Build history of the part. All positions in model axes, mm. Face numbers are marked on the shaded views. A direction names the side the tool comes from. Give positions to 0.01 mm unless a question says otherwise; leave off trailing zeros. Order: outer loops, then holes, each group sorted by start corner. A loop starts at its lowest first (then second) coordinate and runs counter-clockwise, first axis right, second up. Notation, with made-up numbers: (35, 86.5) - (43, 86.5) arc R26 ccw to (43, 123.5) - close; hole circle Ø10 at (-37, -28.5). An arc over 180 degrees is marked (long way). Answer in a Markdown table with one row per item.
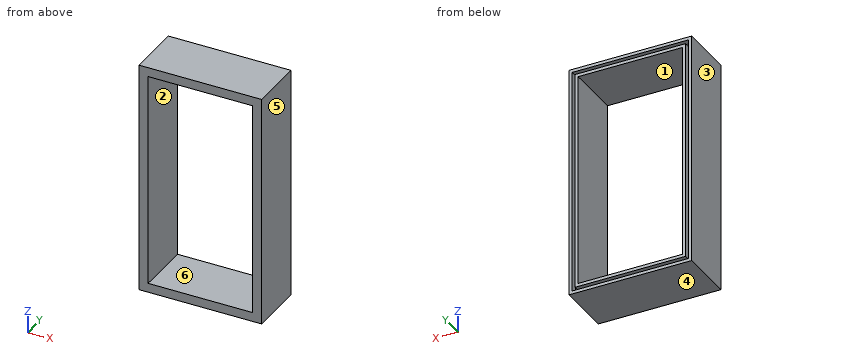
Autodesk Inventor part; units mm, degrees
ref_plane "Work Plane1" through (508, 0, 0) normal (1, 0, 0) x (0, 0, -1)
ref_plane "Work Plane2" through (1016, 0, -965.2) normal (0, 0, -1) x (-1, 0, 0)
ref_plane "YZ Plane" through (0, 0, 0) normal (1, 0, 0) x (0, 1, 0)
sketch "Sketch1" plane through (0, 0, 0) normal (0, 1, 0) x (-1, 0, 0)
  line L0 (0, 0) -> (-1016, 0)
  line L1 (-1016, 0) -> (-1016, -1930.4)
  line L2 (-1016, -1930.4) -> (0, -1930.4)
  line L3 (0, -1930.4) -> (0, 0)
  dimension "d0" = 1016
  dimension "d1" = 1930.4
extrude "Extrusion1" add sketch "Sketch1" along normal blind 457.2
sketch "Sketch8" plane through (0, 457.2, 0) normal (0, 1, 0) x (1, 0, 0)
  line L0 (25.4, 25.4) -> (990.6, 25.4)
  line L1 (990.6, 25.4) -> (990.6, 1905)
  line L2 (990.6, 1905) -> (25.4, 1905)
  line L3 (25.4, 1905) -> (25.4, 25.4)
  line L4 (50.8, 50.8) -> (965.2, 50.8)
  line L5 (965.2, 50.8) -> (965.2, 1879.6)
  line L6 (965.2, 1879.6) -> (50.8, 1879.6)
  line L7 (50.8, 1879.6) -> (50.8, 50.8)
  line L8 (50.8, 965.2) -> (25.4, 965.2)
  line L9 (965.2, 965.2) -> (990.6, 965.2)
  line L10 (508, 1879.6) -> (508, 1905)
  line L11 (508, 50.8) -> (508, 25.4)
  line L12 (508, 25.4) -> (508, 0)
  line L13 (0, 0) -> (1016, 0)
  line L14 (508, 1905) -> (508, 1930.4)
  line L15 (1016, 1930.4) -> (0, 1930.4)
  line L16 (25.4, 965.2) -> (0, 965.2)
  line L17 (0, 1930.4) -> (0, 0)
  line L18 (990.6, 965.2) -> (1016, 965.2)
  line L19 (1016, 0) -> (1016, 1930.4)
  dimension "d13" = 25.4
  dimension "d14" = 25.4
  dimension "d15" = 25.4
  dimension "d16" = 25.4
extrude "Extrusion3" cut sketch "Sketch8" against normal blind 50.8 contours L3 L8 L7 L4 L11 L0 | L11 L4 L5 L9 L1 L0 | L3 L2 L10 L6 L7 L8 | L9 L5 L6 L10 L2 L1
sketch "InnerInset1" plane through (0, 406.4, 0) normal (0, 1, 0) x (1, 0, 0)
  line L0 (25.4, 25.4) -> (25.4, 1905)
  line L1 (50.8, 1879.6) -> (50.8, 50.8)
  line L2 (25.4, 279.4) -> (50.8, 279.4)
  line L3 (50.8, 279.4) -> (50.8, 736.6)
  line L4 (50.8, 736.6) -> (25.4, 736.6)
  line L5 (25.4, 736.6) -> (25.4, 279.4)
  line L6 (990.6, 25.4) -> (25.4, 25.4)
  line L7 (25.4, 1193.8) -> (50.8, 1193.8)
  line L8 (50.8, 1193.8) -> (50.8, 1651)
  line L9 (50.8, 1651) -> (25.4, 1651)
  line L10 (25.4, 1651) -> (25.4, 1193.8)
  line L11 (25.4, 1905) -> (990.6, 1905)
  point P0 (0, 0)
  dimension "d19" = 254
  dimension "d20" = 457.2
  dimension "d21" = 457.2
  dimension "d22" = 254
extrude "Extrusion4" cut sketch "InnerInset1" against normal blind 50.8 contours L0 L4 L1 L2 | L0 L9 L1 L7
ref_plane "Work Plane1" through (508, 0, 0) normal (1, 0, 0) x (0, 0, -1)
mirror "Mirror1" about plane through (508, 0, 0) normal (1, 0, 0) of "Extrusion4"
ref_plane "Work Plane2" through (1016, 0, -965.2) normal (0, 0, -1) x (-1, 0, 0)
sketch "Sketch10" plane through (0, 406.4, 0) normal (0, 1, 0) x (1, 0, 0)
  line L0 (50.8, 50.8) -> (965.2, 50.8)
  line L1 (990.6, 25.4) -> (25.4, 25.4)
  line L2 (203.2, 50.8) -> (355.6, 50.8)
  line L3 (355.6, 50.8) -> (355.6, 25.4)
  line L4 (355.6, 25.4) -> (203.2, 25.4)
  line L5 (203.2, 25.4) -> (203.2, 50.8)
  line L6 (660.4, 50.8) -> (812.8, 50.8)
  line L7 (812.8, 50.8) -> (812.8, 25.4)
  line L8 (812.8, 25.4) -> (660.4, 25.4)
  line L9 (660.4, 25.4) -> (660.4, 50.8)
  line L10 (203.2, 38.1) -> (355.6, 38.1)
  line L11 (660.4, 38.1) -> (812.8, 38.1)
  line L12 (25.4, 25.4) -> (25.4, 1905)
  line L13 (990.6, 1905) -> (990.6, 25.4)
  point P0 (0, 0)
  dimension "d25" = 177.8
  dimension "d26" = 177.8
  dimension "d27" = 152.4
extrude "Extrusion5" cut sketch "Sketch10" against normal blind 50.8 contours L0 L3 L10 L5 | L10 L3 L1 L5 | L0 L7 L11 L9 | L11 L7 L1 L9
mirror "Mirror2" about plane through (1016, 0, -965.2) normal (0, 0, -1) of "Extrusion5"
sketch "Sketch11" plane through (0, 457.2, 0) normal (0, 1, 0) x (1, 0, 0)
  point P0 (0, 0)
sketch "Sketch12" plane through (0, 457.2, 0) normal (0, 1, 0) x (1, 0, 0)
  line L0 (76.2, 1854.2) -> (939.8, 1854.2)
  line L1 (939.8, 1854.2) -> (939.8, 76.2)
  line L2 (939.8, 76.2) -> (76.2, 76.2)
  line L3 (76.2, 76.2) -> (76.2, 1854.2)
  line L4 (76.2, 965.2) -> (50.8, 965.2)
  line L5 (50.8, 1193.8) -> (50.8, 736.6)
  line L6 (939.8, 965.2) -> (965.2, 965.2)
  line L7 (965.2, 736.6) -> (965.2, 1193.8)
  line L8 (508, 1854.2) -> (508, 1879.6)
  line L9 (965.2, 1879.6) -> (50.8, 1879.6)
  line L10 (508, 76.2) -> (508, 50.8)
  line L11 (50.8, 50.8) -> (965.2, 50.8)
  point P0 (0, 0)
  dimension "d30" = 25.4
  dimension "d31" = 25.4
extrude "Extrusion6" cut sketch "Sketch12" against normal blind 609.6
properties part number "rev1 base"
1. Cut at A-A on x = 746. Write the cut outline in (y, z), and give its area (3 significant figures).
Check result:
| item | result |
|---|---|
| outline | (0, -1930.4) - (457.2, -1930.4) - (457.2, -1905) - (355.6, -1905) - (355.6, -1879.6) - (457.2, -1879.6) - (457.2, -1854.2) - (0, -1854.2) - close; (0, -76.2) - (457.2, -76.2) - (457.2, -50.8) - (355.6, -50.8) - (355.6, -25.4) - (457.2, -25.4) - (457.2, 0) - (0, 0) - close |
| area | 64,500 mm² |
2. Drop a flat-ended pin along its axis: P1, Ø12.5, axis at x = 39.5, z = -1409.5, coming from the +Y side. Give the stop position or say it passes through.
Check result:
| item | result |
|---|---|
| P1 | stops at y = 355.6 |
3. Which spindle directions (+Z, -Z, +X, -X, +Y, -Y) get a long thin tool onto all of the face, cutting with end or side? Do the marked faces 5 and 6. Say none if no direction does.
Check result:
| item | result |
|---|---|
| face 5 | +Z, -Z, +X, +Y, -Y |
| face 6 | +Y, -Y |
4. Two-plate mould, pull along Z, no slides. Class the marked faces 1, 2, 3 and 4: +Z half, -Z half, draft (parallel to the pull), parting line (faces both ways), or undercut.
Check result:
| item | result |
|---|---|
| face 1 | undercut |
| face 2 | undercut |
| face 3 | draft |
| face 4 | -Z half |
5. Cut at C-C on y = 216. Write the cut outline in (x, z).
Check result:
| item | result |
|---|---|
| outline | (0, -1930.4) - (1016, -1930.4) - (1016, 0) - (0, 0) - close; hole (76.2, -1854.2) - (939.8, -1854.2) - (939.8, -76.2) - (76.2, -76.2) - close |
6. Cut at B-B on z = -1525.5. Write the cut outline in (x, y).
Check result:
| item | result |
|---|---|
| outline | (0, 0) - (76.2, 0) - (76.2, 457.2) - (50.8, 457.2) - (50.8, 355.6) - (25.4, 355.6) - (25.4, 457.2) - (0, 457.2) - close; (939.8, 0) - (1016, 0) - (1016, 457.2) - (990.6, 457.2) - (990.6, 355.6) - (965.2, 355.6) - (965.2, 457.2) - (939.8, 457.2) - close |
7. Probe line 1 (Z direction, x = 349.5, y = 424.5); line 2 (X direction, y = 432, z = -771); line 3 (X direction, y = 78.5, z = -267). List the from-to ranges inside material, lowest first.
Check result:
| item | result |
|---|---|
| line 1 | z = -1930.4 to -1905, -1879.6 to -1854.2, -76.2 to -50.8, -25.4 to 0 |
| line 2 | x = 0 to 25.4, 50.8 to 76.2, 939.8 to 965.2, 990.6 to 1016 |
| line 3 | x = 0 to 76.2, 939.8 to 1016 |
